```python
from build123d import *

# Parameters (mm, degrees)
SKETCH1_W             = 22.000000096
SKETCH1_H             = 12.7
BOSS_EXTRUDE1_DEPTH   = 6.35
F_8_32_TAPPED_HOLE1_D = 3.4544
SKETCH4_R             = 2.4892
CUT_EXTRUDE1_DEPTH    = 27.184203334


with BuildPart() as part:
    # Sketch1 → Boss-Extrude1 (new, symmetric)
    with BuildSketch(Plane(origin=(0, 0, 0), x_dir=(1, 0, 0), z_dir=(0, 1, 0))):
        with Locations((11.000000048, 6.35)):
            Rectangle(SKETCH1_W, SKETCH1_H)
    extrude(amount=BOSS_EXTRUDE1_DEPTH, both=True)

    # #8-32 Tapped Hole1 (through all)
    with Locations(Plane(origin=(3.000000096, 6.35, -6.35), x_dir=(0, 0, 1), z_dir=(0, 1, 0))):
        with Locations((0, 0), (0, 16)):
            Hole(F_8_32_TAPPED_HOLE1_D / 2)

    # Sketch4 → Cut-Extrude1 (cut, through all)
    with BuildSketch(Plane(origin=(0, 0, -12.7), x_dir=(-1, 0, 0), z_dir=(0, 0, -1))):
        with Locations((-11.000000048, 0)):
            Circle(SKETCH4_R)
    extrude(amount=-CUT_EXTRUDE1_DEPTH, mode=Mode.SUBTRACT)


solid = part.part
```
Can you work these out from the model? Positions are in its coordinate system, mm. Give positions to 0.01 mm unless a question says otherwise; leave off trailing zeros. Order: outer loops, then holes, each group sorted by start corner. A loop starts at its lowest first (then second) coordinate and runs counter-clockwise, first axis right, second up. Notation, with made-up numbers: (35.25, 12) - (49.25, 12) arc R22 ccw to (49.25, 30) - close; hole circle Ø8 at (87, 84). An arc over 180 degrees is marked (long way). Use a Markdown table: item, result. Add a question column.
Q1. Please list where these lines run through material, in increasing order: line 1 along X through (y, z) = (3.5, -6.35); line 2 along Y through (x, z) = (11, -8.75); line 3 along X through (y, z) = (0.5, -7.25).
Q2. If we mould it in two halves opening along Z, with no side actions, what happens to faces 1 (the flat face through (0, 0, -6)), 2 (the cylindrical face through (20.713, -0.089, -6.125)), 3 (the flat face through (8, 0, -12.7))? For each: released by +Z, released by -Z, zero draft, split by the parting line, or undercut.
Q3. If we section it at C-C on z = -6.35: Write out the boundary of the cut face in (x, y), plus the area to 3 significant figures.
Q4. If we section it at A-A on y = 0: Write out the boundary of the cut face in (x, z).
Q5. If we section it at B-B on x = 19: Write out the boundary of the cut face in (y, z).
Q6. If we section it at D-D on y = -5.25: Write out the boundary of the cut face in (x, z).
Answers follow:
| question | item | result |
|---|---|---|
| 1 | line 1 | x = 0 to 1.27, 4.73 to 17.27, 20.73 to 22 |
| 1 | line 2 | y = -6.35 to -2.49, 2.49 to 6.35 |
| 1 | line 3 | x = 0 to 1.53, 4.47 to 8.56, 13.44 to 17.53, 20.47 to 22 |
| 2 | face 1 | zero draft |
| 2 | face 2 | undercut |
| 2 | face 3 | released by -Z |
| 3 | outline | (0, -6.35) - (1.27, -6.35) - (1.27, 6.35) - (0, 6.35) - close; (4.73, -6.35) - (17.27, -6.35) - (17.27, 6.35) - (4.73, 6.35) - close; (20.73, -6.35) - (22, -6.35) - (22, 6.35) - (20.73, 6.35) - close; hole circle Ø4.98 at (11, 0) |
| 3 | area | 172 mm^2 |
| 4 | outline | (0, -12.7) - (8.51, -12.7) - (8.51, 0) - (0, 0) - close; (13.49, -12.7) - (22, -12.7) - (22, 0) - (13.49, 0) - close; hole circle Ø3.45 at (3, -6.35); hole circle Ø3.45 at (19, -6.35) |
| 5 | outline | (-6.35, -12.7) - (6.35, -12.7) - (6.35, -8.08) - (-6.35, -8.08) - close; (-6.35, -4.62) - (6.35, -4.62) - (6.35, 0) - (-6.35, 0) - close |
| 6 | outline | (0, -12.7) - (22, -12.7) - (22, 0) - (0, 0) - close; hole circle Ø3.45 at (3, -6.35); hole circle Ø3.45 at (19, -6.35) |
